Input: part model. Units: mm. Frame: model coordinates. Coordinates: 2 decimals unless noted, no trailing zeros. Loops run counter-clockwise (first coordinate to the right, second up) from the corner with the lowest first, then second, coordinate; pieces in that order, holes last. Notation, with made-up numbers: M 23,-14 L 43,-14 A31 cw 43,18 Z; hole C 46,89.5 d8. An arc over 180 degrees is marked long. Use a Markdown table: item, result. Add a question column.
1. Pin query (flat end, axial travel): pin 1 (1.8 mm diameter, centred on x = -10.5, z = 1.5, fed in from +Y); pin 2 (1.8 mm diameter, centred on y = 10, z = 1.5, fed in from +X); pin 3 (1.1 mm diameter, centred on x = 9, z = 1.5, fed in from -Y). Return the tip coordinate at first contact, or that it passes through.
2. Line query: L1, parallel to X at y = 5, z = 2.25; L2, parallel to X at y = 8.5, z = 2; L3, parallel to X at y = -5.75, z = 0.55. Output: solid intervals per line, ascending. Write a range as [from, to].
3. Section C-C on x = -8.25. Output: boundary loops of the cut face in (y, z).
4. Section B-B on y = 0. Output: boundary loops of the cut face in (x, z), then the cut area to 3 significant figures.
5. Section D-D on z = 0.45. State how many separate pieces and enclosed holes the cut face has, then the cut area to 3 significant figures.
6. Section A-A on x = 0. Output: boundary loops of the cut face in (y, z).
```python
from build123d import *

# Parameters (mm, degrees)
SKETCH_1_R                           = 13
EXTRUDE_1_DEPTH                      = 3.6
SKETCH_2_W                           = 5
SKETCH_2_H                           = 1.6
CUT_EXTRUDE_2_DEPTH                  = 19.733926444
CHAMFER_1_SIZE                       = 0.3
PATTERN_CIRCULAR_1_COUNT             = 20
CHAMFER_1_OF_PATTERN_CIRCULAR_1_SIZE = 0.3


with BuildPart() as part:
    # Sketch 1 → Extrude 1 (new body)
    with BuildSketch(Plane.XY):
        Circle(SKETCH_1_R)
        with BuildLine():
            Line((-2.079062289, 1.8), (2.079062289, 1.8))
            ThreePointArc((2.079062289, 1.8), (2.75, 0), (2.079062289, -1.8))
            Line((2.079062289, -1.8), (-2.079062289, -1.8))
            ThreePointArc((-2.079062289, -1.8), (-2.75, 0), (-2.079062289, 1.8))
        make_face(mode=Mode.SUBTRACT)
    extrude(amount=EXTRUDE_1_DEPTH)

    # Sketch 2 → Cut-Extrude 2 (cut, through all)
    with BuildSketch(Plane.XY):
        with Locations((-9.5, 0)):
            Rectangle(SKETCH_2_W, SKETCH_2_H)
    cut_extrude_2 = extrude(amount=CUT_EXTRUDE_2_DEPTH, mode=Mode.SUBTRACT)

    # Chamfer 1
    chamfer_1_edges = [part.edges().sort_by_distance(p)[0] for p in [
        (-12, 0.8, 1.8),
        (-12, -0.8, 1.8),
        (-7, -0.8, 1.8),
        (-7, 0.8, 1.8),
    ]]
    chamfer(chamfer_1_edges, length=CHAMFER_1_SIZE)

    # Pattern Circular 1: Cut-Extrude 2 ×20 about axis
    pattern_circular_1_axis = Axis((0, 0, 0), (0, 0, 1))
    for i in range(1, PATTERN_CIRCULAR_1_COUNT):
        add(cut_extrude_2.rotate(pattern_circular_1_axis, i * 360 / PATTERN_CIRCULAR_1_COUNT), mode=Mode.SUBTRACT)

    # Chamfer 1 of Pattern Circular 1
    chamfer_1_of_pattern_circular_1_edges = [part.edges().sort_by_distance(p)[0] for p in [
        (-11.659891791, -2.947358719, 1.8),
        (-11.1654646, -4.469049146, 1.8),
        (-6.410182019, -2.923964174, 1.8),
        (-6.90460921, -1.402273748, 1.8),
        (-10.178432134, -6.406209432, 1.8),
        (-9.237975731, -7.700636623, 1.8),
        (-5.192890759, -4.761710362, 1.8),
        (-6.133347162, -3.467283171, 1.8),
        (-7.700636623, -9.237975731, 1.8),
        (-6.406209432, -10.178432134, 1.8),
        (-3.467283171, -6.133347162, 1.8),
        (-4.761710362, -5.192890759, 1.8),
        (-4.469049146, -11.1654646, 1.8),
        (-2.947358719, -11.659891791, 1.8),
        (-1.402273748, -6.90460921, 1.8),
        (-2.923964174, -6.410182019, 1.8),
        (-0.8, -12, 1.8),
        (0.8, -12, 1.8),
        (0.8, -7, 1.8),
        (-0.8, -7, 1.8),
        (2.947358719, -11.659891791, 1.8),
        (4.469049146, -11.1654646, 1.8),
        (2.923964174, -6.410182019, 1.8),
        (1.402273748, -6.90460921, 1.8),
        (6.406209432, -10.178432134, 1.8),
        (7.700636623, -9.237975731, 1.8),
        (4.761710362, -5.192890759, 1.8),
        (3.467283171, -6.133347162, 1.8),
        (9.237975731, -7.700636623, 1.8),
        (10.178432134, -6.406209432, 1.8),
        (6.133347162, -3.467283171, 1.8),
        (5.192890759, -4.761710362, 1.8),
        (11.1654646, -4.469049146, 1.8),
        (11.659891791, -2.947358719, 1.8),
        (6.90460921, -1.402273748, 1.8),
        (6.410182019, -2.923964174, 1.8),
        (12, -0.8, 1.8),
        (12, 0.8, 1.8),
        (7, 0.8, 1.8),
        (7, -0.8, 1.8),
        (11.659891791, 2.947358719, 1.8),
        (11.1654646, 4.469049146, 1.8),
        (6.410182019, 2.923964174, 1.8),
        (6.90460921, 1.402273748, 1.8),
        (10.178432134, 6.406209432, 1.8),
        (9.237975731, 7.700636623, 1.8),
        (5.192890759, 4.761710362, 1.8),
        (6.133347162, 3.467283171, 1.8),
        (7.700636623, 9.237975731, 1.8),
        (6.406209432, 10.178432134, 1.8),
        (3.467283171, 6.133347162, 1.8),
        (4.761710362, 5.192890759, 1.8),
        (4.469049146, 11.1654646, 1.8),
        (2.947358719, 11.659891791, 1.8),
        (1.402273748, 6.90460921, 1.8),
        (2.923964174, 6.410182019, 1.8),
        (0.8, 12, 1.8),
        (-0.8, 12, 1.8),
        (-0.8, 7, 1.8),
        (0.8, 7, 1.8),
        (-2.947358719, 11.659891791, 1.8),
        (-4.469049146, 11.1654646, 1.8),
        (-2.923964174, 6.410182019, 1.8),
        (-1.402273748, 6.90460921, 1.8),
        (-6.406209432, 10.178432134, 1.8),
        (-7.700636623, 9.237975731, 1.8),
        (-4.761710362, 5.192890759, 1.8),
        (-3.467283171, 6.133347162, 1.8),
        (-9.237975731, 7.700636623, 1.8),
        (-10.178432134, 6.406209432, 1.8),
        (-6.133347162, 3.467283171, 1.8),
        (-5.192890759, 4.761710362, 1.8),
        (-11.1654646, 4.469049146, 1.8),
        (-11.659891791, 2.947358719, 1.8),
        (-6.90460921, 1.402273748, 1.8),
        (-6.410182019, 2.923964174, 1.8),
    ]]
    chamfer(chamfer_1_of_pattern_circular_1_edges, length=CHAMFER_1_OF_PATTERN_CIRCULAR_1_SIZE)


solid = part.part
```
Answers below:
| question | item | result |
|---|---|---|
| 1 | pin 1 | stops at y = 8.77 |
| 1 | pin 2 | stops at x = 9.28 |
| 1 | pin 3 | stops at y = -9.88 |
| 2 | L1 | x = [-12, -8.24], [-5.52, 5.52], [8.24, 12] |
| 2 | L2 | x = [-9.84, -7.16], [-5.19, -3.6], [-1.92, -0.8], [0.8, 1.92], [3.6, 5.19], [7.16, 9.84] |
| 2 | L3 | x = [-11.66, -9.28], [-6.55, -5.17], [-3.99, 3.99], [5.17, 6.55], [9.28, 11.66] |
| 3 | outline | M -10.05,0 L -6.98,0 L -6.98,3.6 L -10.05,3.6 Z; M -5.01,0 L -3.52,0 L -3.52,3.6 L -5.01,3.6 Z; M -1.84,0 L -0.8,0 L -0.8,3.6 L -1.84,3.6 Z; M 0.8,0 L 1.84,0 L 1.84,3.6 L 0.8,3.6 Z; M 3.52,0 L 5.01,0 L 5.01,3.6 L 3.52,3.6 Z; M 6.98,0 L 10.05,0 L 10.05,3.6 L 6.98,3.6 Z |
| 4 | outline | M -13,0 L -12,0 L -12,3.6 L -13,3.6 Z; M -7,0 L -2.75,0 L -2.75,3.6 L -7,3.6 Z; M 2.75,0 L 7,0 L 7,3.6 L 2.75,3.6 Z; M 12,0 L 13,0 L 13,3.6 L 12,3.6 Z |
| 4 | area | 37.8 mm² |
| 5 | separate pieces | 1 |
| 5 | enclosed holes | 21 |
| 5 | area | 356 mm² |
| 6 | outline | M -13,0 L -12,0 L -12,3.6 L -13,3.6 Z; M -7,0 L -1.8,0 L -1.8,3.6 L -7,3.6 Z; M 1.8,0 L 7,0 L 7,3.6 L 1.8,3.6 Z; M 12,0 L 13,0 L 13,3.6 L 12,3.6 Z |
